```python
from build123d import *

# Parameters (mm, degrees)
F2_DEPTH = 13
F3_T     = -3
F4_R     = 5.105166
F5_DEPTH = 25


with BuildPart() as f2:
    # F1 (on Top) → F2 (new body)
    with BuildSketch(Plane.XY):
        Polygon((-11.488489, 11.488489), (-16.247177, 0), (-11.488489, -11.488489), (0, -16.247177), (11.488489, -11.488489), (16.247177, 0), (11.488489, 11.488489), (0, 16.247177), align=None)
    extrude(amount=F2_DEPTH)

    # F3
    f3_openings = [f2.faces().sort_by_distance(p)[0] for p in [
        (0, 0, 13),
    ]]
    offset(amount=F3_T, openings=f3_openings)

    # F4 (on Top) → F5 (cut)
    with BuildSketch(Plane.XY):
        Circle(F4_R)
    extrude(amount=F5_DEPTH, mode=Mode.SUBTRACT)


solid = f2.part
```
Geometry: final body of the model. Coordinates: model frame, mm. A direction names the side the tool comes from. Round coordinates to 2 decimals unless told otherwise and drop trailing zeros. Write each loop counter-clockwise with the first axis right and the second up, starting at its lowest first coordinate (ties: lowest second). Pieces come first, ordered by that corner, then holes. Notation, with made-up numbers: (-20.75, 19.25) -> (35.25, 19.25) arc R22 cw to (35.25, 57.25) -> close; hole circle Ø11 at (52.25, 1.25). An arc over 180 degrees is marked (long way). Return JSON: item names as keys, results as strings.
Q1. Section D-D on y = -13.5. Return the cut outline in (x, z).
From the geometry:
{"outline": "(-6.63, 0) -> (6.63, 0) -> (6.63, 13) -> (-6.63, 13) -> close"}
Q2. Mould query, pull axis X, two halves, no side actions, for faces 1 (the flat face through (-5.825, -13.835, 6.409)), 2 (the flat face through (-4, 4, 0)), 3 (the flat face through (11.07, -4.66, 7.93)). Classes: +X half, -X half, draft (parallel to the pull), parting line (faces both ways), or undercut.
From the geometry:
{"face 1": "-X half", "face 2": "draft", "face 3": "undercut"}
Q3. Ray query, line 1 (X direction, y = 0, z = 1.65); line 2 (Z direction, x = -5, y = 5). Return the intervals inside material, ascending.
From the geometry:
{"line 1": "-16.25 to -5.11, 5.11 to 16.25", "line 2": "0 to 3"}
Q4. Section C-C on x = 7. Return the cut outline in (y, z), and give its area (3 significant figures).
From the geometry:
{"outline": "(-13.35, 0) -> (13.35, 0) -> (13.35, 13) -> (10.1, 13) -> (10.1, 3) -> (-10.1, 3) -> (-10.1, 13) -> (-13.35, 13) -> close", "area": "145 mm2"}
Q5. Set-up query: faces 4 (the flat face through (5.825, 13.835, 6.409)), 5 (the flat face through (4.66, 11.07, 7.93)). Return all of +Z, -Z, +X, -X, +Y, -Y with unobstructed straight access to the full face (end or side cutting, diameter ignored); none if empty.
From the geometry:
{"face 4": "+Z, -Z, +X, +Y", "face 5": "+Z"}
Q6. First-contact query: pin 1 Ø4 at (x, z) = (5.5, 1.5) entering from -Y; pin 2 Ø8 at (x, y) = (-1, -1.5) entering from +Z; pin 3 Ø2 at (x, z) = (-3, 2) entering from -Y. Flat tips, straight axial feed; report the tip coordinate or a pass-through.
From the geometry:
{"pin 1": "y = -14.8", "pin 2": "z = 3", "pin 3": "y = -15.42"}
Q7. Section B-B on z = 7.5. Return the cut outline in (x, y).
From the geometry:
{"outline": "(-16.25, 0) -> (-11.49, -11.49) -> (0, -16.25) -> (11.49, -11.49) -> (16.25, 0) -> (11.49, 11.49) -> (0, 16.25) -> (-11.49, 11.49) -> close; hole (-13, 0) -> (-9.19, -9.19) -> (0, -13) -> (9.19, -9.19) -> (13, 0) -> (9.19, 9.19) -> (0, 13) -> (-9.19, 9.19) -> close"}
Q8. Section A-A on x = 2. Return the cut outline in (y, z), and give its area (3 significant figures).
From the geometry:
{"outline": "(-15.42, 0) -> (-4.7, 0) -> (-4.7, 3) -> (-12.17, 3) -> (-12.17, 13) -> (-15.42, 13) -> close; (4.7, 0) -> (15.42, 0) -> (15.42, 13) -> (12.17, 13) -> (12.17, 3) -> (4.7, 3) -> close", "area": "129 mm2"}
